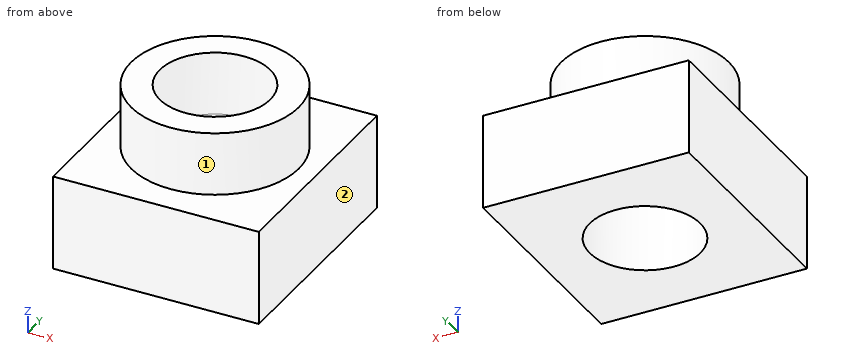
```python
from build123d import *

# Parameters (mm, degrees)
F0_W      = 82.344018
F0_H      = 90.373024
F1_DEPTH  = 38.1
F2_R      = 33.560103
F2_R_2    = 22.134941
F3_DEPTH  = 25.4
F3_FACE_R = 22.134941
F4_DEPTH  = 127


with BuildPart() as f1:
    # F0 (on Top) → F1 (new body)
    with BuildSketch(Plane.XY):
        Rectangle(F0_W, F0_H)
    extrude(amount=F1_DEPTH)

    # F2 (on face) → F3 (join)
    with BuildSketch(Plane.XY.offset(38.1)):
        Circle(F2_R)
        Circle(F2_R_2, mode=Mode.SUBTRACT)
    extrude(amount=F3_DEPTH)

    # F3_face (on face) → F4 (cut)
    with BuildSketch(Plane.XY.offset(38.1)):
        Circle(F3_FACE_R)
    extrude(amount=-F4_DEPTH, mode=Mode.SUBTRACT)


solid = f1.part
```
The model under review builds one solid part; all positions refer to its coordinate system, in mm. Face numbers are marked on the shaded views. A direction names the side the tool comes from. Round coordinates to 2 decimals unless told otherwise and drop trailing zeros. Loops run counter-clockwise (first coordinate to the right, second up) from the corner with the lowest first, then second, coordinate; pieces in that order, holes last. Notation, with made-up numbers: (19, 82) -> (36, 82) arc R21 cw to (36, 87) -> close; hole circle Ø10 at (-18, -15.75). An arc over 180 degrees is marked (long way). Answer in a Markdown table with one row per item.
1) Consider section D-D, the plane y = -23.5. Write out the cut boundary in (x, z).
Taken from the geometry:
| item | result |
|---|---|
| outline | (-41.17, 0) -> (41.17, 0) -> (41.17, 38.1) -> (23.96, 38.1) -> (23.96, 63.5) -> (-23.96, 63.5) -> (-23.96, 38.1) -> (-41.17, 38.1) -> close |
2) Consider section B-B, the plane x = 0. Write out the cut boundary in (y, z).
Taken from the geometry:
| item | result |
|---|---|
| outline | (-45.19, 0) -> (-22.13, 0) -> (-22.13, 63.5) -> (-33.56, 63.5) -> (-33.56, 38.1) -> (-45.19, 38.1) -> close; (22.13, 0) -> (45.19, 0) -> (45.19, 38.1) -> (33.56, 38.1) -> (33.56, 63.5) -> (22.13, 63.5) -> close |
3) Consider section A-A, the plane y = 0. Write out the cut boundary in (x, z).
Taken from the geometry:
| item | result |
|---|---|
| outline | (-41.17, 0) -> (-22.13, 0) -> (-22.13, 63.5) -> (-33.56, 63.5) -> (-33.56, 38.1) -> (-41.17, 38.1) -> close; (22.13, 0) -> (41.17, 0) -> (41.17, 38.1) -> (33.56, 38.1) -> (33.56, 63.5) -> (22.13, 63.5) -> close |
4) Tool access review of the marked faces 1 and 2: name each direction out of +Z, -Z, +X, -X, +Y, -Y from which nothing blocks a thin tool from reaching the whole face with its end or side.
Taken from the geometry:
| item | result |
|---|---|
| face 1 | +Z |
| face 2 | +Z, -Z, +X, +Y, -Y |
5) For pin 1 Ø1.5 at (x, z) = (-14, 51) entering from +Y, flat-tipped, find the tip position at first contact; note if it passes through.
Taken from the geometry:
| item | result |
|---|---|
| pin 1 | stops at y = 30.83 |
6) Consider section C-C, the plane z = 36.5. Write out the cut boundary in (x, y).
Taken from the geometry:
| item | result |
|---|---|
| outline | (-41.17, -45.19) -> (41.17, -45.19) -> (41.17, 45.19) -> (-41.17, 45.19) -> close; hole circle Ø44.27 at (0, 0) |
7) Wall thickness on line 1 along Y through (x, z) = (0, 12); line 2 along Y through (x, z) = (0, 43.75); line 3 along Z through (x, y) = (26.5, 37.5): over which ranges is each line inside the solid? List them lowest first.
Taken from the geometry:
| item | result |
|---|---|
| line 1 | y = -45.19 to -22.13, 22.13 to 45.19 |
| line 2 | y = -33.56 to -22.13, 22.13 to 33.56 |
| line 3 | z = 0 to 38.1 |
